For this review, take the finished solid that the model builds, in its own axes (mm). A direction names the side the tool comes from. Coordinates: 2 decimals unless noted, no trailing zeros. Write each loop counter-clockwise with the first axis right and the second up, starting at its lowest first coordinate (ties: lowest second). Pieces come first, ordered by that corner, then holes.
1) We need section C-C on z = 1.75. Write out the cut boundary in (x, y).
2) We need section D-D on y = -4.75. Write out the cut boundary in (x, z).
3) To check wall thickness, follow line 1 along Y through (x, z) = (0, 5.85); line 2 along Y through (x, z) = (0, -0.1); line 3 along Z through (x, y) = (3.5, 3). State the ranges of each line that lie inside material, in increasing order.
4) Insertion check: P1, Ø2, axis at y = 1.5, z = 2, coming from the -X side; P2, Ø1.5, axis at y = 2.5, z = 1.5, coming from the +X side. Each pin has a flat end and moves straight along its axis. Give the tip position at first contact, or say it passes through.
5) We need section A-A on x = 0. Write out the cut boundary in (y, z), then the cut area to 3 significant figures.
6) For faces 1 (the face through (-4, -2, 5.5)), 2 (the face through (1, 3, -0.5)), list the 3-axis set-ups (+Z, -Z, +X, -X, +Y, -Y) from which the entire face can be reached by the end or side of a thin tool; tool diameter is ignored.
from build123d import *

# Parameters (mm, degrees)
ESBO_O1_R                = 3.5
ESBO_O1_R_2              = 3
RESSALTO_EXTRUS_O1_DEPTH = 5.5
ESBO_O2_R                = 3.5
ESBO_O2_R_2              = 3
RESSALTO_EXTRUS_O2_DEPTH = 0.5
ESBO_O3_R                = 5.5
ESBO_O3_R_2              = 3
RESSALTO_EXTRUS_O4_DEPTH = 0.5
FILETE1_R                = 0.5
CHANFRO1_SIZE            = 0.3
CHANFRO1_SIZE2           = 0.173205081


with BuildPart() as part:
    # Esboço1 → Ressalto-extrusão1 (new body)
    with BuildSketch(Plane.XY):
        Circle(ESBO_O1_R)
        Circle(ESBO_O1_R_2, mode=Mode.SUBTRACT)
    extrude(amount=RESSALTO_EXTRUS_O1_DEPTH)

    # Esboço2 → Ressalto-extrusão2 (add)
    with BuildSketch(Plane(origin=(0, 0, 0), x_dir=(-1, 0, 0), z_dir=(0, 0, -1))):
        Circle(ESBO_O2_R)
        Circle(ESBO_O2_R_2, mode=Mode.SUBTRACT)
    extrude(amount=RESSALTO_EXTRUS_O2_DEPTH)

    # Esboço3 → Ressalto-extrusão4 (add)
    with BuildSketch(Plane.XY.offset(5.5)):
        Circle(ESBO_O3_R)
        Circle(ESBO_O3_R_2, mode=Mode.SUBTRACT)
    extrude(amount=RESSALTO_EXTRUS_O4_DEPTH)

    # Filete1
    filete1_edges = [part.edges().sort_by_distance(p)[0] for p in [
        (-3.5, 0, 5.5),
    ]]
    fillet(filete1_edges, radius=FILETE1_R)

    # Chanfro1
    chanfro1_edges = [part.edges().sort_by_distance(p)[0] for p in [
        (3.5, 0, -0.5),
    ]]
    chanfro1_side = [part.faces().sort_by_distance(p)[0] for p in [
        (3.5, 0, -0.25),
    ]]
    chamfer(chanfro1_edges, length=CHANFRO1_SIZE, length2=CHANFRO1_SIZE2, reference=chanfro1_side[0])


solid = part.part
Result:
1. outline: circle Ø7 at (0, 0); hole circle Ø6 at (0, 0)
2. outline: (-2.77, 5.5) - (2.77, 5.5) - (2.77, 6) - (-2.77, 6) - close
3. line 1: y = -5.5 to -3, 3 to 5.5
3. line 2: y = -3.5 to -3, 3 to 3.5
3. line 3: z = 5.5 to 6
4. P1: stops at x = -3.46
4. P2: stops at x = 3.03
5. outline: (-5.5, 5.5) - (-4, 5.5) arc R0.5 cw to (-3.5, 5) - (-3.5, -0.2) - (-3.33, -0.5) - (-3, -0.5) - (-3, 6) - (-5.5, 6) - close; (3, -0.5) - (3.33, -0.5) - (3.5, -0.2) - (3.5, 5) arc R0.5 cw to (4, 5.5) - (5.5, 5.5) - (5.5, 6) - (3, 6) - close
5. area: 8.56 mm2
6. face 1: -Z
6. face 2: -Z, +X, -X, +Y, -Y
